from build123d import *

# Parameters (mm, degrees)
SKETCH1_W           = 85
SKETCH1_H           = 55
BOSS_EXTRUDE1_DEPTH = 25
SKETCH2_W           = 55
SKETCH2_H           = 26
CUT_EXTRUDE1_DEPTH  = 10.5
FILLET1_R           = 1.55
SKETCH3_W           = 67
SKETCH3_H           = 38
SKETCH3_W_2         = 62
SKETCH3_H_2         = 33
CUT_EXTRUDE2_DEPTH  = 0.25
FILLET2_R           = 1.55
SKETCH5_R           = 2.025
CUT_EXTRUDE4_DEPTH  = 26


with BuildPart() as part:
    # Sketch1 → Boss-Extrude1 (new body)
    with BuildSketch(Plane(origin=(0, 0, 0), x_dir=(1, 0, 0), z_dir=(0, 1, 0))):
        with Locations((42.5, 27.5)):
            Rectangle(SKETCH1_W, SKETCH1_H)
    extrude(amount=BOSS_EXTRUDE1_DEPTH)

    # Sketch2 → Cut-Extrude1 (cut)
    with BuildSketch(Plane(origin=(0, 25, 0), x_dir=(1, 0, 0), z_dir=(0, 1, 0))):
        with Locations((42.5, 27.5)):
            Rectangle(SKETCH2_W, SKETCH2_H)
    extrude(amount=-CUT_EXTRUDE1_DEPTH, mode=Mode.SUBTRACT)

    # Fillet1
    fillet1_edges = [part.edges().sort_by_distance(p)[0] for p in [
        (15, 19.75, -14.5),
        (15, 19.75, -40.5),
        (70, 19.75, -40.5),
        (70, 19.75, -14.5),
        (0, 12.5, -55),
        (85, 12.5, -55),
        (85, 12.5, 0),
        (0, 12.5, 0),
    ]]
    fillet(fillet1_edges, radius=FILLET1_R)

    # Sketch3 → Cut-Extrude2 (cut)
    with BuildSketch(Plane(origin=(0, 25, 0), x_dir=(1, 0, 0), z_dir=(0, 1, 0))):
        with Locations((42.5, 27.5)):
            Rectangle(SKETCH3_W, SKETCH3_H)
        with Locations((42.5, 27.5)):
            Rectangle(SKETCH3_W_2, SKETCH3_H_2, mode=Mode.SUBTRACT)
    extrude(amount=-CUT_EXTRUDE2_DEPTH, mode=Mode.SUBTRACT)

    # Fillet2
    fillet2_edges = [part.edges().sort_by_distance(p)[0] for p in [
        (9, 24.875, -8.5),
        (9, 24.875, -46.5),
        (76, 24.875, -46.5),
        (76, 24.875, -8.5),
        (11.5, 24.875, -44),
        (73.5, 24.875, -44),
        (73.5, 24.875, -11),
        (11.5, 24.875, -11),
    ]]
    fillet(fillet2_edges, radius=FILLET2_R)

    # Sketch5 → Cut-Extrude4 (cut, through all)
    with BuildSketch(Plane(origin=(0, 25, 0), x_dir=(1, 0, 0), z_dir=(0, 1, 0))):
        with Locations((5, 42.45)):
            Circle(SKETCH5_R)
        with Locations((5, 12.55)):
            Circle(SKETCH5_R)
        with Locations((13.05, 4.5)):
            Circle(SKETCH5_R)
        with Locations((71.95, 4.5)):
            Circle(SKETCH5_R)
        with Locations((24.83, 4.5)):
            Circle(SKETCH5_R)
        with Locations((36.61, 4.5)):
            Circle(SKETCH5_R)
        with Locations((48.39, 4.5)):
            Circle(SKETCH5_R)
        with Locations((60.17, 4.5)):
            Circle(SKETCH5_R)
        with Locations((5, 32.483333333)):
            Circle(SKETCH5_R)
        with Locations((5, 22.516666667)):
            Circle(SKETCH5_R)
        with Locations((80, 42.45)):
            Circle(SKETCH5_R)
        with Locations((80, 12.55)):
            Circle(SKETCH5_R)
        with Locations((80, 22.516666667)):
            Circle(SKETCH5_R)
        with Locations((80, 32.483333333)):
            Circle(SKETCH5_R)
        with Locations((13.05, 50.5)):
            Circle(SKETCH5_R)
        with Locations((24.83, 50.5)):
            Circle(SKETCH5_R)
        with Locations((36.61, 50.5)):
            Circle(SKETCH5_R)
        with Locations((48.39, 50.5)):
            Circle(SKETCH5_R)
        with Locations((60.17, 50.5)):
            Circle(SKETCH5_R)
        with Locations((71.95, 50.5)):
            Circle(SKETCH5_R)
    extrude(amount=-CUT_EXTRUDE4_DEPTH, mode=Mode.SUBTRACT)


solid = part.part
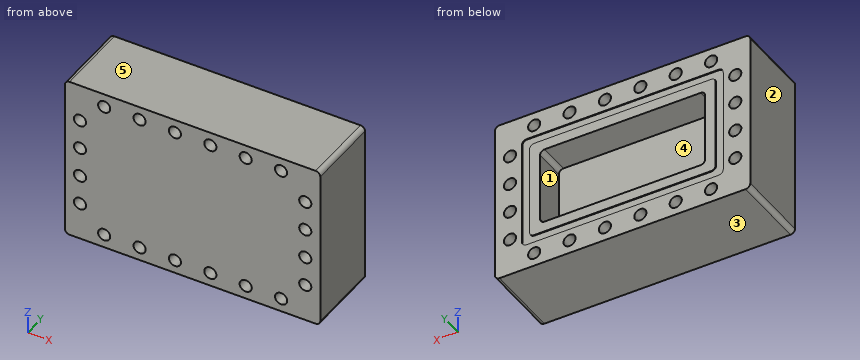
Work out the finished part from the listing and answer in its coordinate system (mm). Face numbers are marked on the shaded views. A direction names the side the tool comes from. Give positions to 0.01 mm unless a question says otherwise; leave off trailing zeros. Loops run counter-clockwise (first coordinate to the right, second up) from the corner with the lowest first, then second, coordinate; pieces in that order, holes last. Notation, with made-up numbers: (72.25, 12.25) - (126.25, 12.25) arc R12 ccw to (126.25, 34.25) - close; hole circle Ø3 at (80.25, -13.75). An arc over 180 degrees is marked (long way). Answer in a Markdown table with one row per item. Add a question column.
Q1. The part is cut by section C-C (z = -4.5). Determine the outline of the cut face in (x, y) (3 decimals).
Q2. The part is cut by section D-D (y = 2). State how many separate pieces and enclosed holes the cut face has, and give its area (3 significant figures).
Q3. Determine the mould class of the marked faces 1, 2 and 3 for opening direction Z: released by +Z, released by -Z, zero draft, split by the parting line, or undercut.
Q4. The part is cut by section A-A (x = 5). Determine the outline of the cut face in (y, z) (3 decimals).
Q5. This flat-tipped pin is pushed along its axis until it touches: P1, Ø3.5, axis at x = 48.39, z = -4.5, coming from the +Y side. Where does it stop, or does it pass through?
Q6. A tool of negligible diameter and unlimited length cuts with its end or side. For the marked faces 4 and 5, from which of +Z, -Z, +X, -X, +Y, -Y can it reach the whole face along a straight path? Write none if from no direction.
Q7. Consider line 1 along Z through (x, y) = (5, 7.5) (3 decimals); line 2 along Z through (x, y) = (48.39, 16) (3 decimals); line 3 along Z through (x, y) = (25, 2.5). Determine where each line is inside the solid, lowest interval first.
Q8. The part is cut by section B-B (x = 24.83). Determine the outline of the cut face in (y, z) (3 decimals).
Solution:
| question | item | result |
|---|---|---|
| 1 | outline | (0, 0) - (11.025, 0) - (11.025, 25) - (0, 25) - close; (15.075, 0) - (22.805, 0) - (22.805, 25) - (15.075, 25) - close; (26.855, 0) - (34.585, 0) - (34.585, 25) - (26.855, 25) - close; (38.635, 0) - (46.365, 0) - (46.365, 25) - (38.635, 25) - close; (50.415, 0) - (58.145, 0) - (58.145, 25) - (50.415, 25) - close; (62.195, 0) - (69.925, 0) - (69.925, 25) - (62.195, 25) - close; (73.975, 0) - (85, 0) - (85, 25) - (73.975, 25) - close |
| 2 | separate pieces | 1 |
| 2 | enclosed holes | 20 |
| 2 | area | 4,420 mm² |
| 3 | face 1 | undercut |
| 3 | face 2 | zero draft |
| 3 | face 3 | released by -Z |
| 4 | outline | (0, -55) - (25, -55) - (25, -44.475) - (0, -44.475) - close; (0, -40.425) - (25, -40.425) - (25, -34.508) - (0, -34.508) - close; (0, -30.458) - (25, -30.458) - (25, -24.542) - (0, -24.542) - close; (0, -20.492) - (25, -20.492) - (25, -14.575) - (0, -14.575) - close; (0, -10.525) - (25, -10.525) - (25, 0) - (0, 0) - close |
| 5 | P1 | passes through |
| 6 | face 4 | +Y |
| 6 | face 5 | +Z, +X, -X, +Y, -Y |
| 7 | line 1 | z = -55 to -44.475, -40.425 to -34.508, -30.458 to -24.542, -20.492 to -14.575, -10.525 to 0 |
| 7 | line 2 | z = -55 to -52.525, -48.475 to -40.5, -14.5 to -6.525, -2.475 to 0 |
| 7 | line 3 | z = -55 to -52.52, -48.48 to -6.52, -2.48 to 0 |
| 8 | outline | (0, -55) - (25, -55) - (25, -52.525) - (0, -52.525) - close; (0, -48.475) - (25, -48.475) - (25, -46.5) - (24.75, -46.5) - (24.75, -44) - (25, -44) - (25, -40.5) - (14.5, -40.5) - (14.5, -14.5) - (25, -14.5) - (25, -11) - (24.75, -11) - (24.75, -8.5) - (25, -8.5) - (25, -6.525) - (0, -6.525) - close; (0, -2.475) - (25, -2.475) - (25, 0) - (0, 0) - close |
